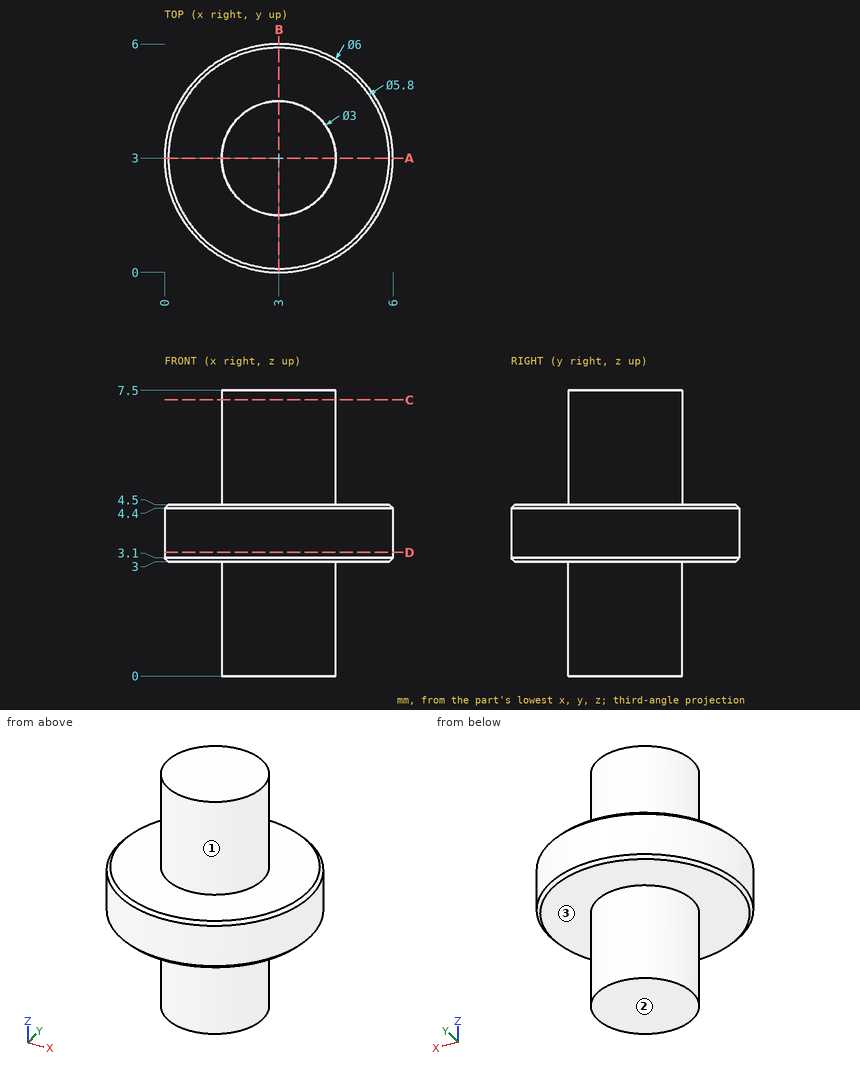
Can you work these out from the drawing? Everything is in mm from the part's minimum corner. A direction names the side the tool comes from. Give positions to 0.01 mm unless a question says otherwise; leave off trailing zeros. Loops run counter-clockwise (first coordinate to the right, second up) from the corner with the lowest first, then second, coordinate; pieces in that order, holes last. Notation, with made-up numbers: (76.5, -13) -> (85.5, -13) arc R14 ccw to (85.5, -5) -> close; hole circle Ø8 at (62, 69.25). An arc over 180 degrees is marked (long way). Return JSON: item names as keys, results as strings.
Item 1: I need wall thicknesses on L1, parallel to Z at x = 0.4, y = 1.9; L2, parallel to X at y = 4.05, z = 5.75; L3, parallel to Y at x = 1.6, z = 3.25. Which ranges of each line are inside material? Lowest first, please. Write a range as from..to.
Geometry results:
{"L1": "z = 3..4.5", "L2": "x = 1.93..4.07", "L3": "y = 0.35..5.65"}
Item 2: If we section it at C-C on z = 7.25: List the corners of the cut face in (x, y) for me, plus the area to 3 significant figures.
Geometry results:
{"outline": "circle Ø3 at (3, 3)", "area": "7.07 mm²"}
Item 3: If we section it at A-A on y = 3: List the corners of the cut face in (x, z) for me, plus the area to 3 significant figures.
Geometry results:
{"outline": "(0, 3.1) -> (0.1, 3) -> (1.5, 3) -> (1.5, 0) -> (4.5, 0) -> (4.5, 3) -> (5.9, 3) -> (6, 3.1) -> (6, 4.4) -> (5.9, 4.5) -> (4.5, 4.5) -> (4.5, 7.5) -> (1.5, 7.5) -> (1.5, 4.5) -> (0.1, 4.5) -> (0, 4.4) -> close", "area": "27.0 mm²"}
Item 4: Which directions (+Z, -Z, +X, -X, +Y, -Y) give clear straight access to the entire face, cutting with the end or side of a thin tool? Please do the marked faces 1, 2 and 3.
Geometry results:
{"face 1": "+Z", "face 2": "-Z, +X, -X, +Y, -Y", "face 3": "-Z"}
Item 5: If we section it at D-D on z = 3.25: List the corners of the cut face in (x, y) for me.
Geometry results:
{"outline": "circle Ø6 at (3, 3)"}
